Work out the finished part from the listing and answer in its coordinate system (mm). A direction names the side the tool comes from. Give positions to 0.01 mm unless a question says otherwise; leave off trailing zeros. Loops run counter-clockwise (first coordinate to the right, second up) from the corner with the lowest first, then second, coordinate; pieces in that order, holes last. Notation, with made-up numbers: M -15.5,-28 L 8.5,-28 A30 ccw 8.5,11 Z; hole C 53.25,87.25 d11. An arc over 180 degrees is marked long. Write item = value, one per line. Start each with the question number.
1. Section A-A on x = 282 is taken. Determine the outline of the cut face in (y, z) (3 decimals), plus the area to 3 significant figures.
2. Flat-ended cylindrical pins translate along their axes: pin 1 Ø7 at (y, z) = (1, 3.5) entering from -X; pin 2 Ø5 at (x, z) = (151, 3) entering from +Y; pin 3 Ø6 at (x, y) = (186.5, 0) entering from -Z (3 decimals); pin 4 Ø4 at (y, z) = (4, 4) entering from -X. Find the tip coordinate at first contact, or state that the pin passes through.
3. For faces 1 (the face through (0, 0, 0)), 2 (the face through (258.6, -2.2, 2)), 3 (the face through (82.7, -2.2, 2)), 4 (the face through (52.7, -2.2, 2)), 5 (the face through (172.373, -1.507, -6.785)), determine the directions among +Z, -Z, +X, -X, +Y, -Y from which every point of the face is accessible in a straight line to the end or side of a thin tool.
4. Consider L1, parallel to X at y = -2.25, z = 3.25; L2, parallel to Z at x = 154, y = 0.25; L3, parallel to Y at x = 226, z = 2. Determine where each line is inside the solid, lowest interval first. Write a range as [from, to].
```python
from build123d import *

# Parameters (mm, degrees)
ESQUISSE2_W                  = 16.4
ESQUISSE2_H                  = 2.788709481
ESQUISSE2_W_2                = 8.697698695
ESQUISSE2_H_2                = 2.899232898
ENL_V_MAT_EXTRU_1_DEPTH      = 7.95
ENL_V_MAT_EXTRU_1_DEPTH_BACK = 7.95
CHANFREIN1_SIZE              = 0.25


with BuildPart() as part:
    # Esquisse1 → Révolution1 (revolve)
    with BuildSketch(Plane.XY):
        Polygon((0, 0), (0, 2.975), (1.7, 2.975), (1.7, 2.35), (3.4, 2.35), (3.4, 2.975), (45.65, 2.975), (45.65, 2.35), (47.35, 2.35), (47.35, 2.975), (57.85, 2.975), (57.85, 6.95), (74.55, 6.95), (74.55, 2.975), (90.55, 2.975), (90.55, 6.95), (107.25, 6.95), (107.25, 2.975), (126.05, 2.975), (126.05, 6.95), (140, 6.95), (140, 2.975), (165.3, 2.975), (165.3, 6.95), (179.25, 6.95), (179.25, 2.975), (198.05, 2.975), (198.05, 6.95), (214.75, 6.95), (214.75, 2.975), (230.75, 2.975), (230.75, 6.95), (247.45, 6.95), (247.45, 2.975), (269.45, 2.975), (269.45, 2.35), (271.15, 2.35), (271.15, 2.975), (300.15, 2.975), (300.15, 2.35), (301.85, 2.35), (301.85, 2.975), (303.55, 2.975), (303.55, 0), align=None)
    revolve(axis=Axis((0, 0, 0), (1, 0, 0)))

    # Esquisse2 → Enlèv. mat.-Extru.1 (cut, two sides)
    with BuildSketch(Plane(origin=(0, 0, 0), x_dir=(1, 0, 0), z_dir=(0, 1, 0))) as enl_v_mat_extru_1_sk:
        with Locations((8.2, 3.399354741)):
            Rectangle(ESQUISSE2_W, ESQUISSE2_H)
        with Locations((301.498849348, -3.454616449)):
            Rectangle(ESQUISSE2_W_2, ESQUISSE2_H_2)
    extrude(amount=ENL_V_MAT_EXTRU_1_DEPTH, mode=Mode.SUBTRACT)
    extrude(enl_v_mat_extru_1_sk.sketch, amount=-ENL_V_MAT_EXTRU_1_DEPTH_BACK, mode=Mode.SUBTRACT)

    # Chanfrein1
    chanfrein1_edges = [part.edges().sort_by_distance(p)[0] for p in [
        (0, 0, 2.975),
        (303.55, 0, -2.975),
    ]]
    chamfer(chanfrein1_edges, length=CHANFREIN1_SIZE)


solid = part.part
```
Verdict:
q1.outline = C 0,0 d5.95
q1.area = 27.8 mm2
q2.pin_1 = 0
q2.pin_2 = 2.93
q2.pin_3 = -2.975
q2.pin_4 = 57.85
q3.face_1 = +Z, -Z, -X, +Y, -Y
q3.face_2 = +X
q3.face_3 = none
q3.face_4 = -X
q3.face_5 = +X, -X
q4.L1 = [57.85, 74.55], [90.55, 107.25], [126.05, 140], [165.3, 179.25], [198.05, 214.75], [230.75, 247.45]
q4.L2 = [-2.96, 2.96]
q4.L3 = [-2.2, 2.2]
